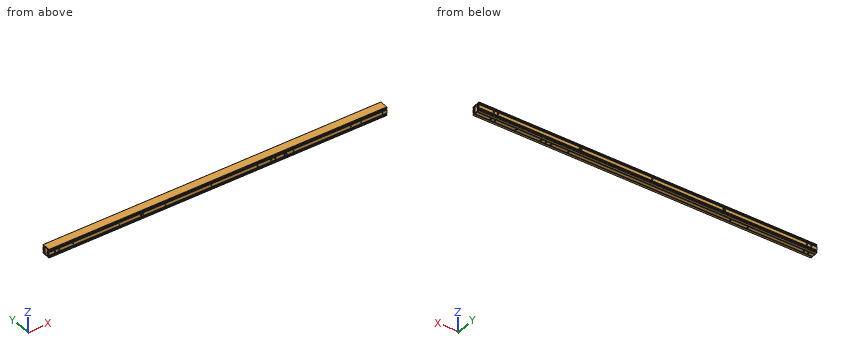
from build123d import *

# Parameters (mm, degrees)
SKETCH_1_W             = 23.5
SKETCH_1_H             = 12
EXTRUDE_1_DEPTH        = 586
HOLE_WIZARD_M6_1_D     = 5
HOLE_WIZARD_M6_1_DEPTH = 15
HOLE_WIZARD_M6_1_TIP   = 1.502151548
HOLE_WIZARD_M6_2_D     = 5
HOLE_WIZARD_M6_2_DEPTH = 15
HOLE_WIZARD_M6_2_TIP   = 1.502151548
HOLE_WIZARD_M6_3_D     = 5
HOLE_WIZARD_M6_3_DEPTH = 15
HOLE_WIZARD_M6_3_TIP   = 1.502151548
SKETCH_10_R            = 5.05
CUT_EXTRUDE_1_DEPTH    = 587.959112716
HOLE_WIZARD_M4_1_D     = 3.3
HOLE_WIZARD_M4_1_DEPTH = 10.1
HOLE_WIZARD_M4_1_TIP   = 0.991420021
HOLE_WIZARD_M4_2_D     = 3.3
HOLE_WIZARD_M4_2_DEPTH = 10.1
HOLE_WIZARD_M4_2_TIP   = 0.991420021
HOLE_WIZARD_M4_3_D     = 3.3
HOLE_WIZARD_M4_3_DEPTH = 10.1
HOLE_WIZARD_M4_3_TIP   = 0.991420021
HOLE_WIZARD_M6_4_D     = 5
HOLE_WIZARD_M6_4_DEPTH = 15
HOLE_WIZARD_M6_4_TIP   = 1.502151548


with BuildPart() as part:
    # 草图1 → 凸台-拉伸1 (new, symmetric)
    with BuildSketch(Plane(origin=(0, 0, 0), x_dir=(0, 0, -1), z_dir=(1, 0, 0))):
        with BuildLine():
            Line((-14, 15), (-11.5, 15))
            Line((-11.5, 15), (-11.5, 13.5))
            Line((-11.5, 13.5), (-11.4, 13.5))
            ThreePointArc((-11.4, 13.5), (-11.117157288, 13.382842712), (-11, 13.1))
            Line((-11, 13.1), (-11, 12))
            Line((-11, 12), (-9.5, 12))
            Line((-9.5, 12), (-9.5, 15))
            Line((-9.5, 15), (-8, 15))
            Line((-8, 15), (-8, 12.5))
            Line((-8, 12.5), (-5, 12.5))
            Line((-5, 12.5), (-5, 15))
            Line((-5, 15), (5, 15))
            Line((5, 15), (5, 12.5))
            Line((5, 12.5), (8, 12.5))
            Line((8, 12.5), (8, 15))
            Line((8, 15), (9.5, 15))
            Line((9.5, 15), (9.5, 12))
            Line((9.5, 12), (11, 12))
            Line((11, 12), (11, 13.1))
            ThreePointArc((11, 13.1), (11.117157288, 13.382842712), (11.4, 13.5))
            Line((11.4, 13.5), (11.5, 13.5))
            Line((11.5, 13.5), (11.5, 15))
            Line((11.5, 15), (14, 15))
            ThreePointArc((14, 15), (14.707106781, 14.707106781), (15, 14))
            Line((15, 14), (15, 8))
            Line((15, 8), (12.5, 8))
            Line((12.5, 8), (12.5, 5))
            Line((12.5, 5), (15, 5))
            Line((15, 5), (15, -5))
            Line((15, -5), (12.5, -5))
            Line((12.5, -5), (12.5, -8))
            Line((12.5, -8), (15, -8))
            Line((15, -8), (15, -14))
            ThreePointArc((15, -14), (14.707106781, -14.707106781), (14, -15))
            Line((14, -15), (11.5, -15))
            Line((11.5, -15), (11.5, -13.5))
            Line((11.5, -13.5), (11.4, -13.5))
            ThreePointArc((11.4, -13.5), (11.117157288, -13.382842712), (11, -13.1))
            Line((11, -13.1), (11, -12))
            Line((11, -12), (9.5, -12))
            Line((9.5, -12), (9.5, -15))
            Line((9.5, -15), (8, -15))
            Line((8, -15), (8, -12.5))
            Line((8, -12.5), (5, -12.5))
            Line((5, -12.5), (5, -15))
            Line((5, -15), (-5, -15))
            Line((-5, -15), (-5, -12.5))
            Line((-5, -12.5), (-8, -12.5))
            Line((-8, -12.5), (-8, -15))
            Line((-8, -15), (-9.5, -15))
            Line((-9.5, -15), (-9.5, -12))
            Line((-9.5, -12), (-11, -12))
            Line((-11, -12), (-11, -13.1))
            ThreePointArc((-11, -13.1), (-11.117157288, -13.382842712), (-11.4, -13.5))
            Line((-11.4, -13.5), (-11.5, -13.5))
            Line((-11.5, -13.5), (-11.5, -15))
            Line((-11.5, -15), (-14, -15))
            ThreePointArc((-14, -15), (-14.707106781, -14.707106781), (-15, -14))
            Line((-15, -14), (-15, 14))
            ThreePointArc((-15, 14), (-14.707106781, 14.707106781), (-14, 15))
        make_face()
        with BuildLine():
            Line((12, -10.5), (12, -8.5))
            ThreePointArc((12, -8.5), (11.853553391, -8.146446609), (11.5, -8))
            Line((11.5, -8), (-11.5, -8))
            ThreePointArc((-11.5, -8), (-11.853553391, -8.146446609), (-12, -8.5))
            Line((-12, -8.5), (-12, -10.5))
            ThreePointArc((-12, -10.5), (-11.853553391, -10.853553391), (-11.5, -11))
            Line((-11.5, -11), (11.5, -11))
            ThreePointArc((11.5, -11), (11.853553391, -10.853553391), (12, -10.5))
        make_face(mode=Mode.SUBTRACT)
        with BuildLine():
            Line((-11.5, 11), (11.5, 11))
            ThreePointArc((11.5, 11), (11.853553391, 10.853553391), (12, 10.5))
            Line((12, 10.5), (12, 8.5))
            ThreePointArc((12, 8.5), (11.853553391, 8.146446609), (11.5, 8))
            Line((11.5, 8), (-11.5, 8))
            ThreePointArc((-11.5, 8), (-11.853553391, 8.146446609), (-12, 8.5))
            Line((-12, 8.5), (-12, 10.5))
            ThreePointArc((-12, 10.5), (-11.853553391, 10.853553391), (-11.5, 11))
        make_face(mode=Mode.SUBTRACT)
        Rectangle(SKETCH_1_W, SKETCH_1_H, mode=Mode.SUBTRACT)
    extrude(amount=EXTRUDE_1_DEPTH, both=True)

    # M6 螺纹孔1
    with Locations(Plane.XZ.offset(15)):
        with Locations((-566, 0), (-551, 0), (184, 0), (199, 0)):
            Hole(HOLE_WIZARD_M6_1_D / 2, depth=HOLE_WIZARD_M6_1_DEPTH)
            with Locations((0, 0, -(HOLE_WIZARD_M6_1_DEPTH + HOLE_WIZARD_M6_1_TIP / 2))):  # 118° drill point
                Cone(0, HOLE_WIZARD_M6_1_D / 2, HOLE_WIZARD_M6_1_TIP, mode=Mode.SUBTRACT)

    # M6 螺纹孔2
    with Locations(Plane(origin=(0, 0, -15), x_dir=(-1, 0, 0), z_dir=(0, 0, -1))):
        with Locations((566, 0), (551, 0), (-521, 0), (-536, 0), (-448, 0), (-361, 0), (-344, 0)):
            Hole(HOLE_WIZARD_M6_2_D / 2, depth=HOLE_WIZARD_M6_2_DEPTH)
            with Locations((0, 0, -(HOLE_WIZARD_M6_2_DEPTH + HOLE_WIZARD_M6_2_TIP / 2))):  # 118° drill point
                Cone(0, HOLE_WIZARD_M6_2_D / 2, HOLE_WIZARD_M6_2_TIP, mode=Mode.SUBTRACT)

    # M6 螺纹孔3
    with Locations(Plane(origin=(0, 15, 0), x_dir=(-1, 0, 0), z_dir=(0, 1, 0))):
        with Locations((-536, 0), (-521, 0), (551, 0), (566, 0), (14, 0)):
            Hole(HOLE_WIZARD_M6_3_D / 2, depth=HOLE_WIZARD_M6_3_DEPTH)
            with Locations((0, 0, -(HOLE_WIZARD_M6_3_DEPTH + HOLE_WIZARD_M6_3_TIP / 2))):  # 118° drill point
                Cone(0, HOLE_WIZARD_M6_3_D / 2, HOLE_WIZARD_M6_3_TIP, mode=Mode.SUBTRACT)

    # 草图10 → 切除-拉伸1 (cut, through all)
    with BuildSketch(Plane(origin=(0, 15, 0), x_dir=(1, 0, 0), z_dir=(0, 1, 0))):
        with Locations(Location((234, 0, 0), (0, 0, 270))):
            Circle(SKETCH_10_R)
        with Locations(Location((-264, 0, 0), (0, 0, 270))):
            Circle(SKETCH_10_R)
    extrude(amount=-CUT_EXTRUDE_1_DEPTH, mode=Mode.SUBTRACT)

    # M4 螺纹孔1
    with Locations(Plane.XZ.offset(15)):
        with Locations((137, 0), (-23, 0), (-183, 0), (-343, 0), (-503, 0)):
            Hole(HOLE_WIZARD_M4_1_D / 2, depth=HOLE_WIZARD_M4_1_DEPTH)
            with Locations((0, 0, -(HOLE_WIZARD_M4_1_DEPTH + HOLE_WIZARD_M4_1_TIP / 2))):  # 118° drill point
                Cone(0, HOLE_WIZARD_M4_1_D / 2, HOLE_WIZARD_M4_1_TIP, mode=Mode.SUBTRACT)

    # M4 螺纹孔2
    with Locations(Plane.XZ.offset(15)):
        with Locations((461, 0), (261, 0)):
            Hole(HOLE_WIZARD_M4_2_D / 2, depth=HOLE_WIZARD_M4_2_DEPTH)
            with Locations((0, 0, -(HOLE_WIZARD_M4_2_DEPTH + HOLE_WIZARD_M4_2_TIP / 2))):  # 118° drill point
                Cone(0, HOLE_WIZARD_M4_2_D / 2, HOLE_WIZARD_M4_2_TIP, mode=Mode.SUBTRACT)

    # M4 螺纹孔3
    with Locations(Plane.XZ.offset(15)):
        with Locations((571, 0), (496, 0)):
            Hole(HOLE_WIZARD_M4_3_D / 2, depth=HOLE_WIZARD_M4_3_DEPTH)
            with Locations((0, 0, -(HOLE_WIZARD_M4_3_DEPTH + HOLE_WIZARD_M4_3_TIP / 2))):  # 118° drill point
                Cone(0, HOLE_WIZARD_M4_3_D / 2, HOLE_WIZARD_M4_3_TIP, mode=Mode.SUBTRACT)

    # M6 螺纹孔4
    with Locations(Plane(origin=(0, 0, -15), x_dir=(-1, 0, 0), z_dir=(0, 0, -1))):
        with Locations((-326, 0), (-266, 0), (296, 0), (356, 0)):
            Hole(HOLE_WIZARD_M6_4_D / 2, depth=HOLE_WIZARD_M6_4_DEPTH)
            with Locations((0, 0, -(HOLE_WIZARD_M6_4_DEPTH + HOLE_WIZARD_M6_4_TIP / 2))):  # 118° drill point
                Cone(0, HOLE_WIZARD_M6_4_D / 2, HOLE_WIZARD_M6_4_TIP, mode=Mode.SUBTRACT)


solid = part.part
Verification items for the finished model (mm, model axes). Coordinates: 2 decimals unless noted, no trailing zeros. One line per item, written item: value. Start each with the question number.
Item 1: Thickness scan on probe 1 along Y at (x, z) = (-403.5, 3.25); probe 2 along Y at (x, z) = (143.5, -7); probe 3 along Z at (x, y) = (184, -12.65). Record the ranges inside material, lowest first.
Item 2: Depth check by flat-ended pin: P1, Ø1, axis at x = 346.5, z = 6.5, coming from the -Y side. Enter the tip coordinate at first touch or a pass-through.
Item 3: Sectioned sample at A-A on x = 479.5. Give the number of separate pieces and of enclosed holes in the cut face, then the cut area to 3 significant figures.
Calculated:
1. probe 1: -15 to -11, -8 to -6, 6 to 8, 11 to 15
1. probe 2: -12.5 to -11, -8 to -6, 6 to 8, 11 to 12.5
1. probe 3: -15 to -11, -9.5 to -8, -5 to -2.5, 2.5 to 5, 8 to 9.5, 11 to 15
2. P1: y = -12.5
3. separate pieces: 1
3. enclosed holes: 3
3. area: 407 mm^2
